from build123d import *

# Parameters (mm, degrees)
SKETCH086_W     = 106
SKETCH086_H     = 22
PAD005_DEPTH    = 3
SKETCH087_R     = 1.25
POCKET003_DEPTH = 3
FILLET005_R     = 8
SKETCH088_R     = 1.65
POCKET004_DEPTH = 3


with BuildPart() as part:
    # Sketch086 → Pad005 (new body)
    with BuildSketch(Plane.XY):
        with Locations((0.609999, 10.86)):
            Rectangle(SKETCH086_W, SKETCH086_H)
    extrude(amount=PAD005_DEPTH)

    # Sketch087 → Pocket003 (cut)
    with BuildSketch(Plane.XY.offset(3)):
        with Locations((-38.549999, 10.83)):
            Circle(SKETCH087_R)
        with Locations((39.800001, 10.823599)):
            Circle(SKETCH087_R)
    extrude(amount=-POCKET003_DEPTH, mode=Mode.SUBTRACT)

    # Fillet005
    fillet005_edges = [part.edges().sort_by_distance(p)[0] for p in [
        (-52.390001, 21.86, 1.5),
        (-52.390001, -0.14, 1.5),
        (53.609999, 21.86, 1.5),
        (53.609999, -0.14, 1.5),
    ]]
    fillet(fillet005_edges, radius=FILLET005_R)

    # Sketch088 (on Face5 of Fillet005) → Pocket004 (cut)
    with BuildSketch(Plane.XY.offset(3)):
        with Locations((-49.240092, 10.86)):
            Circle(SKETCH088_R)
        with Locations((50.460174, 10.86)):
            Circle(SKETCH088_R)
    extrude(amount=-POCKET004_DEPTH, mode=Mode.SUBTRACT)


with BuildPart() as part_1:
    # Body008 placement: moved
    add(part.part.moved(Location((46.37, -59.87, 16))))


with BuildPart() as part_2:
    # Clone placement: moved
    add(part_1.part.moved(Location((8.020001, 36.01, -19))))


solid = part_2.part
Can you work these out from the model? Positions are in its coordinate system, mm. Give positions to 0.01 mm unless a question says otherwise; leave off trailing zeros. Order: outer loops, then holes, each group sorted by start corner. A loop starts at its lowest first (then second) coordinate and runs counter-clockwise, first axis right, second up. Notation, with made-up numbers: M 71,55 L 106,55 A26 ccw 106,90 Z; hole C 0,24 d9. An arc over 180 degrees is marked long. One line per item, written item: value.
Item 1: Please list where these lines run through material, in increasing order: line 1 (X direction, y = -13.25, z = -0.2); line 2 (X direction, y = -12.25, z = -1.25); line 3 (X direction, y = -16.5, z = -1.5).
Verdict:
line 1: 2 to 3.52, 6.78 to 14.61, 17.07 to 92.96, 95.42 to 103.22, 106.48 to 108
line 2: 2 to 3.68, 6.62 to 14.86, 16.82 to 93.22, 95.16 to 103.38, 106.32 to 108
line 3: 2.02 to 107.98
Item 2: If we section it at B-B on y = -4.5: Write out the boundary of the cut face in (x, z), and give its area (3 significant figures).
Verdict:
outline: M 4.19,-3 L 105.81,-3 L 105.81,0 L 4.19,0 Z
area: 305 mm2
Item 3: If we section it at A-A on z = -2.05: Write out the boundary of the cut face in (x, y).
Verdict:
outline: M 2,-16 A8 ccw 10,-24 L 100,-24 A8 ccw 108,-16 L 108,-10 A8 ccw 100,-2 L 10,-2 A8 ccw 2,-10 Z; hole C 5.15,-13 d3.3; hole C 15.84,-13.03 d2.5; hole C 94.19,-13.04 d2.5; hole C 104.85,-13 d3.3
Item 4: For pin 1 (4 mm diameter, centred on x = 104.85, y = -13, fed in from +Z); pin 2 (2 mm diameter, centred on x = 15.84, y = -13.03, fed in from -Z); pin 3 (1 mm diameter, centred on y = -17.5, z = -1, fed in from -X), each with a flat end and sliding along its axis, tell me the tip position at first contact or that it passes through.
Verdict:
pin 1: z = 0
pin 2: through
pin 3: x = 2.06
Item 5: If we mould it in two halves opening along Y, with no side actions, what happens to faces 1 (the face through (2, -13, -2)), 2 (the face through (95.38, -12.66, -1.48)), 3 (the face through (105.594, -21.719, -1.479))? For each: pulls with the +Y half, pulls with the -Y half, needs draft (parallel to the pull), parting line crosses it, or undercut.
Verdict:
face 1: needs draft
face 2: undercut
face 3: pulls with the -Y half
